from build123d import *

# Parameters (mm, degrees)
SKETCH001_W  = 200
SKETCH001_H  = 70
PAD_DEPTH    = 2
FILLET_R     = 8
SKETCH_R     = 1.75
SKETCH_W     = 15
SKETCH_H     = 2
SKETCH_W_2   = 2
SKETCH_H_2   = 15
POCKET_DEPTH = 2


with BuildPart() as part:
    # Sketch001 → Pad (new body)
    with BuildSketch(Plane.XY):
        with Locations((100, 35)):
            Rectangle(SKETCH001_W, SKETCH001_H)
    extrude(amount=PAD_DEPTH)

    # Fillet
    fillet_edges = [part.edges().sort_by_distance(p)[0] for p in [
        (0, 70, 1),
        (200, 70, 1),
        (0, 0, 1),
        (200, 0, 1),
    ]]
    fillet(fillet_edges, radius=FILLET_R)

    # Sketch → Pocket (cut)
    with BuildSketch(Plane.XY):
        with Locations((20, 55)):
            Circle(SKETCH_R)
        with Locations((20, 15)):
            Circle(SKETCH_R)
        with Locations((180, 55)):
            Circle(SKETCH_R)
        with Locations((180, 15)):
            Circle(SKETCH_R)
        with Locations((105.5, 37)):
            Circle(SKETCH_R)
        with Locations((46.5, 66)):
            Rectangle(SKETCH_W, SKETCH_H)
        with Locations((46.5, 4)):
            Rectangle(SKETCH_W, SKETCH_H)
        with Locations((153.5, 66)):
            Rectangle(SKETCH_W, SKETCH_H)
        with Locations((153.5, 4)):
            Rectangle(SKETCH_W, SKETCH_H)
        with Locations((9, 35)):
            Rectangle(SKETCH_W_2, SKETCH_H_2)
        with Locations((191, 35)):
            Rectangle(SKETCH_W_2, SKETCH_H_2)
    extrude(amount=POCKET_DEPTH, mode=Mode.SUBTRACT)


solid = part.part
Here's how the part is built. I have some questions about the finished solid (model axes, mm). Round coordinates to 2 decimals unless told otherwise and drop trailing zeros. Loops run counter-clockwise (first coordinate to the right, second up) from the corner with the lowest first, then second, coordinate; pieces in that order, holes last.
1. If we section it at C-C on y = 55: Write out the boundary of the cut face in (x, z), plus the area to 3 significant figures.
Answer list:
outline: (0, 0) - (18.25, 0) - (18.25, 2) - (0, 2) - close; (21.75, 0) - (178.25, 0) - (178.25, 2) - (21.75, 2) - close; (181.75, 0) - (200, 0) - (200, 2) - (181.75, 2) - close
area: 386 mm2
2. If we section it at B-B on x = 105.5: Write out the boundary of the cut face in (y, z).
Answer list:
outline: (0, 0) - (35.25, 0) - (35.25, 2) - (0, 2) - close; (38.75, 0) - (70, 0) - (70, 2) - (38.75, 2) - close
3. If we section it at D-D on x = 20: Write out the boundary of the cut face in (y, z).
Answer list:
outline: (0, 0) - (13.25, 0) - (13.25, 2) - (0, 2) - close; (16.75, 0) - (53.25, 0) - (53.25, 2) - (16.75, 2) - close; (56.75, 0) - (70, 0) - (70, 2) - (56.75, 2) - close
4. We'd pull the mould along Y, two halves only. Please class faces 1 (the face through (181.669, 55.526, 0.986)), 2 (the face through (99, 35, 2)), 3 (the face through (2.281, 67.594, 1.014)): +Y half, -Y half, draft (parallel to the pull), parting line (faces both ways), or undercut.
Answer list:
face 1: undercut
face 2: draft
face 3: +Y half
5. If we section it at A-A on y = 37: Write out the boundary of the cut face in (x, z), plus the area to 3 significant figures.
Answer list:
outline: (0, 0) - (8, 0) - (8, 2) - (0, 2) - close; (10, 0) - (103.75, 0) - (103.75, 2) - (10, 2) - close; (107.25, 0) - (190, 0) - (190, 2) - (107.25, 2) - close; (192, 0) - (200, 0) - (200, 2) - (192, 2) - close
area: 385 mm2
6. For P1, Ø2, axis at x = 172, y = 44, coming from the -Z side; P2, Ø0.6, axis at y = 65.5, z = 1, coming from the -X side; P3, Ø1, axis at y = 65.5, z = 1, coming from the +X side; P4, Ø0.6, axis at y = 4, z = 0.5, coming from the -X side, each with a flat end and sliding along its axis, tell me the tip position at first contact or that it passes through.
Answer list:
P1: stops at z = 0
P2: stops at x = 0.67
P3: stops at x = 199.42
P4: stops at x = 0.91
7. If I drill on line 1 along Y through (x, z) = (20, 1.3); line 2 along Y through (x, z) = (41.5, 0.65); line 3 along Y through (x, z) = (105.5, 0.9), over which ranges is the centre line in solid material (lowest first)?
Answer list:
line 1: y = 0 to 13.25, 16.75 to 53.25, 56.75 to 70
line 2: y = 0 to 3, 5 to 65, 67 to 70
line 3: y = 0 to 35.25, 38.75 to 70
